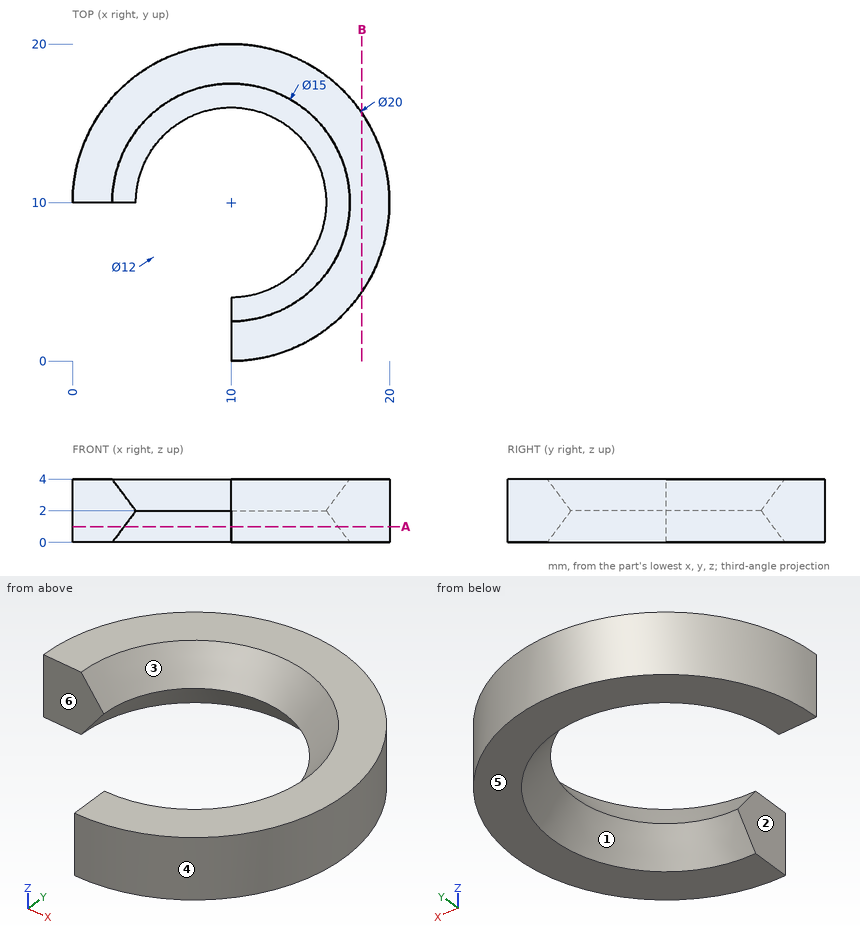
Input: dimensioned drawing with shaded views. Units: mm. Origin: part minimum x, y, z. A direction names the side the tool comes from. Give positions to 0.01 mm unless a question says otherwise; leave off trailing zeros. Write each loop counter-clockwise with the first axis right and the second up, starting at its lowest first coordinate (ties: lowest second). Pieces come first, ordered by that corner, then holes. Notation, with made-up numbers: M 22,83 L 39,83 A19 ccw 39,117 Z; hole C 31.25,39.5 d8. An arc over 180 degrees is marked long. Return JSON: item names as keys, results as strings. Group by question number.
1) Pin query (flat end, axial travel): P1, Ø1, axis at x = 12, z = 3.5, coming from the +Y side; P2, Ø1.5, axis at x = 15.5, z = 3.5, coming from the -Y side. Return the tip coordinate at first contact, or that it passes through.
2) Cut plane B-B, the plane x = 18.25. Output: boundary loops of the cut face in (y, z), plus the area to 3 significant figures.
3) Material intervals for line 1 along Y through (x, z) = (13.5, 2.65); line 2 along X through (y, z) = (13.5, 2.2); line 3 along X through (y, z) = (15.5, 2.65), sorted ascending. Write a range as [from, to].
4) Pull-direction query (Y, two-part tool) for the marked faces 1, 2, 3 and 4; classes: pulls with the +Y half, pulls with the -Y half, needs draft (parallel to the pull), parting line crosses it, or undercut.
5) Set-up query: the marked faces 5 and 6. Return all of +Z, -Z, +X, -X, +Y, -Y with unobstructed straight access to the full face (end or side cutting, diameter ignored); none if empty.
6) Cut plane A-A, the plane z = 1. Output: boundary loops of the cut face in (x, y), plus the area to 3 significant figures.
Recorded:
{
 "1": {"P1": "stops at y = 19.89", "P2": "stops at y = 1.2"},
 "2": {"outline": "M 4.35,0 L 15.65,0 L 15.65,4 L 4.35,4 Z", "area": "45.2 mm²"},
 "3": {"line 1": "y = [0.63, 4.54], [15.46, 19.37]", "line 2": "x = [0.63, 4.94], [15.06, 19.37]", "line 3": "x = [1.65, 6.56], [13.44, 18.35]"},
 "4": {"face 1": "undercut", "face 2": "needs draft", "face 3": "undercut", "face 4": "parting line crosses it"},
 "5": {"face 5": "-Z, +X, -X, +Y, -Y", "face 6": "+Z, -Z, -X, -Y"},
 "6": {"outline": "M 0,10 L 3.25,10 A6.75 cw long 10,3.25 L 10,0 A10 ccw long Z", "area": "128 mm²"}
}
